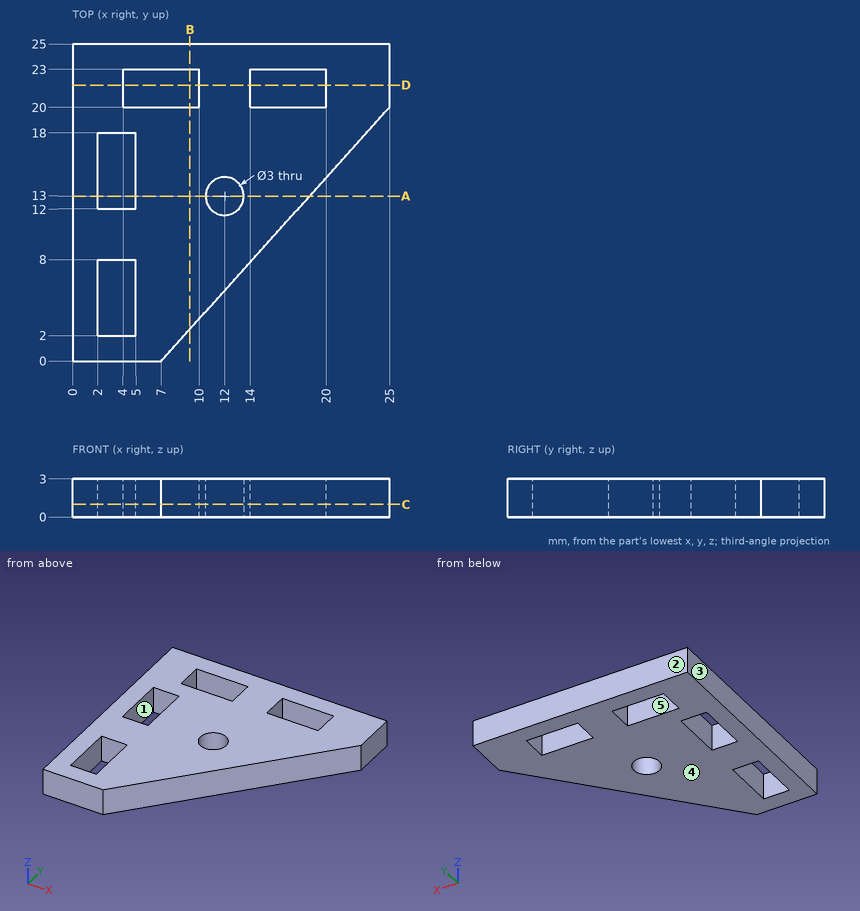
Here's the drawing with two shaded views (mm, measured from the low corner). I have some questions. A direction names the side the tool comes from. Round coordinates to 2 decimals unless told otherwise and drop trailing zeros. Order: outer loops, then holes, each group sorted by start corner. A loop starts at its lowest first (then second) coordinate and runs counter-clockwise, first axis right, second up. Notation, with made-up numbers: (-20.75, 59) -> (5.25, 59) arc R12 cw to (5.25, 74) -> close; hole circle Ø5 at (89, 72.5). An arc over 180 degrees is marked (long way). Use a Markdown table: item, result. Add a question column.
(1) Suppose I cut it at B-B, the plane x = 9.25. Please give me the cut outline in (y, z), and give its area (3 significant figures).
(2) Suppose I cut it at A-A, the plane y = 13. Please give me the cut outline in (x, z), and give its area (3 significant figures).
(3) For the marked faces 4 and 5, which set-ups out of +Z, -Z, +X, -X, +Y, -Y let a thin tool reach every point of the face, with its end or its side?
(4) Suppose I cut it at C-C, the plane z = 1. Please give me the cut outline in (x, y), and give its area (3 significant figures).
(5) Suppose I cut it at D-D, the plane y = 21.75. Please give me the cut outline in (x, z), and give its area (3 significant figures).
(6) If we mould it in two halves opening along Y, with no side actions, what happens to the marked faces 1, 2 and 3? For each: released by +Y, released by -Y, zero draft, split by the parting line, or undercut.
(7) For pin 1 Ø2 at (x, y) = (18, 17.5) entering from -Z; pin 2 Ø0.9 at (x, z) = (18.5, 2) entering from -Y, each with a flat end and sliding along its axis, tell me the tip position at first contact or that it passes through.
(8) I need wall thicknesses on line 1 along X through (y, z) = (22.25, 2.4); line 2 along Y through (x, z) = (3, 2.7); line 3 along Y through (x, z) = (6, 2.2). Which ranges of each line are inside material? Lowest first, please.
Verdict:
| question | item | result |
|---|---|---|
| 1 | outline | (2.5, 0) -> (20, 0) -> (20, 3) -> (2.5, 3) -> close; (23, 0) -> (25, 0) -> (25, 3) -> (23, 3) -> close |
| 1 | area | 58.5 mm2 |
| 2 | outline | (0, 0) -> (2, 0) -> (2, 3) -> (0, 3) -> close; (5, 0) -> (10.5, 0) -> (10.5, 3) -> (5, 3) -> close; (13.5, 0) -> (18.7, 0) -> (18.7, 3) -> (13.5, 3) -> close |
| 2 | area | 38.1 mm2 |
| 3 | face 4 | -Z, +X, -X, +Y, -Y |
| 3 | face 5 | +Z, -Z |
| 4 | outline | (0, 0) -> (7, 0) -> (25, 20) -> (25, 25) -> (0, 25) -> close; hole (2, 2) -> (5, 2) -> (5, 8) -> (2, 8) -> close; hole (2, 12) -> (5, 12) -> (5, 18) -> (2, 18) -> close; hole (4, 20) -> (10, 20) -> (10, 23) -> (4, 23) -> close; hole circle Ø3 at (12, 13); hole (14, 20) -> (20, 20) -> (20, 23) -> (14, 23) -> close |
| 4 | area | 366 mm2 |
| 5 | outline | (0, 0) -> (4, 0) -> (4, 3) -> (0, 3) -> close; (10, 0) -> (14, 0) -> (14, 3) -> (10, 3) -> close; (20, 0) -> (25, 0) -> (25, 3) -> (20, 3) -> close |
| 5 | area | 39.0 mm2 |
| 6 | face 1 | undercut |
| 6 | face 2 | released by +Y |
| 6 | face 3 | zero draft |
| 7 | pin 1 | z = 0 |
| 7 | pin 2 | y = 12.28 |
| 8 | line 1 | 0 to 4, 10 to 14, 20 to 25 |
| 8 | line 2 | 0 to 2, 8 to 12, 18 to 25 |
| 8 | line 3 | 0 to 20, 23 to 25 |
